Autodesk Inventor part; units mm, degrees
ref_plane "YZ Plane" through (0, 0, 0) normal (1, 0, 0) x (0, 1, 0)
ref_plane "XZ Plane" through (0, 0, 0) normal (0, 1, 0) x (-1, 0, 0)
ref_plane "XY Plane" through (0, 0, 0) normal (0, 0, 1) x (1, 0, 0)
sketch "Sketch1" plane through (0, 0, 0) normal (0, 0, 1) x (1, 0, 0)
  line L0 (-30, -85) -> (30, -85)
  line L1 (30, -85) -> (30, 85)
  line L2 (30, 85) -> (-30, 85)
  line L3 (-30, 85) -> (-30, -85)
  line L4 (-30, -85) -> (30, 85) construction
  line L5 (30, -85) -> (-30, 85) construction
  line L6 (-19, 19) -> (19, 19)
  line L7 (19, 19) -> (19, -19)
  line L8 (19, -19) -> (-19, -19)
  line L9 (-19, -19) -> (-19, 19)
  line L10 (-19, 19) -> (19, -19) construction
  line L11 (19, 19) -> (-19, -19) construction
  circle A0 centre (19, 19) radius 1.5875
  circle A1 centre (19, 19) radius 3
  circle A2 centre (-19, 19) radius 3
  circle A3 centre (-19, 19) radius 1.5875
  circle A4 centre (-19, -19) radius 3
  circle A5 centre (-19, -19) radius 1.5875
  circle A6 centre (19, -19) radius 3
  circle A7 centre (19, -19) radius 1.5875
  circle A8 centre (19, -35) radius 3
  circle A9 centre (19, -35) radius 1.5875
  circle A10 centre (-19, -35) radius 1.5875
  circle A11 centre (-19, -35) radius 3
  circle A12 centre (-19, -73) radius 3
  circle A13 centre (-19, -73) radius 1.5875
  circle A14 centre (19, -73) radius 3
  circle A15 centre (19, -73) radius 1.5875
  circle A16 centre (19, 73) radius 3
  circle A17 centre (19, 73) radius 1.5875
  circle A18 centre (-19, 73) radius 1.5875
  circle A19 centre (-19, 73) radius 3
  circle A20 centre (-19, 35) radius 3
  circle A21 centre (-19, 35) radius 1.5875
  circle A22 centre (19, 35) radius 3
  circle A23 centre (19, 35) radius 1.5875
  circle A24 centre (19, 19) radius 3
  circle A25 centre (19, 19) radius 1.5875
  circle A26 centre (-19, 19) radius 1.5875
  circle A27 centre (-19, 19) radius 3
  circle A28 centre (-19, -19) radius 3
  circle A29 centre (-19, -19) radius 1.5875
  circle A30 centre (19, -19) radius 3
  circle A31 centre (19, -19) radius 1.5875
  point P0 (0, 0)
  dimension "d0" = 170
  dimension "d1" = 60
  dimension "d2" = 38
  dimension "d3" = 38
  dimension "d6" = 6
  dimension "d7" = 3.175
  dimension "d10" = 360
  dimension "d14" = 54
  dimension "d17" = 54
extrude "Extrusion1" add sketch "Sketch1" along normal blind 3.2 contours L3 L2 L1 L0 | L6 A1 L7 A6 L8 A4 L9 A2
extrude "Extrusion2" add sketch "Sketch1" along normal blind 5 contours A3 L9 A2 L6 | L6 A2 L9 A3 | A1 L7 A0 L6 | L6 A0 L7 A1 | A4 L8 A5 L9 | L9 A5 L8 A4 | A6 L8 A7 L7 | L7 A7 L8 A6 | A8 | A11 | A12 | A14 | A16 | A19 | A20 | A22
sketch "Sketch2" plane through (0, 0, 3.2) normal (0, 0, 1) x (1, 0, 0)
  line L0 (-15.4, 31.4) -> (-0.6, 31.4)
  line L1 (-0.6, 31.4) -> (-0.6, 26.4)
  line L2 (-0.6, 26.4) -> (-15.4, 26.4)
  line L3 (-15.4, 26.4) -> (-15.4, 31.4)
  circle A0 centre (-19, 35) radius 1.5875
  line L4 (-19, 35) -> (-15.4, 31.4)
  line L5 (-19, 35) -> (-14, 35)
  line L6 (-30, 85) -> (-30, -85)
  line L7 (-30, 0) -> (-30, 23)
  line L8 (-15.4, -22.6) -> (-0.6, -22.6)
  line L9 (-0.6, -22.6) -> (-0.6, -27.6)
  line L10 (-0.6, -27.6) -> (-15.4, -27.6)
  line L11 (-15.4, -27.6) -> (-15.4, -22.6)
  line L12 (-15.4, -76.6) -> (-0.6, -76.6)
  line L13 (-0.6, -76.6) -> (-0.6, -81.6)
  line L14 (-0.6, -81.6) -> (-15.4, -81.6)
  line L15 (-15.4, -81.6) -> (-15.4, -76.6)
  line L16 (-14.2, 31.4) -> (-15.4, 30.2)
  line L17 (-8, 26.4) -> (-8, 31.4)
  line L18 (-0.6, 28.9) -> (-8, 28.9)
  line L19 (-1.8, 31.4) -> (-0.6, 30.2)
  line L20 (-14.2, 26.4) -> (-15.4, 27.6)
  line L21 (-1.8, 26.4) -> (-0.6, 27.6)
  line L22 (-14.2, -22.6) -> (-15.4, -23.8)
  line L23 (-1.8, -22.6) -> (-0.6, -23.8)
  line L24 (-1.8, -27.6) -> (-0.6, -26.4)
  line L25 (-14.2, -27.6) -> (-15.4, -26.4)
  line L26 (-14.2, -76.6) -> (-15.4, -77.8)
  line L27 (-1.8, -76.6) -> (-0.6, -77.8)
  line L28 (-1.8, -81.6) -> (-0.6, -80.4)
  line L29 (-14.2, -81.6) -> (-15.4, -80.4)
  point P0 (0, 0)
  point P1 (-15.4, -80.4)
  point P2 (-0.6, -80.4)
  point P3 (-0.6, -77.8)
  point P4 (-15.4, -77.8)
  point P5 (-15.4, -26.4)
  point P6 (-0.6, -26.4)
  point P7 (-0.6, -23.8)
  point P8 (-15.4, -23.8)
  point P9 (-15.4, 27.6)
  point P10 (-0.6, 27.6)
  point P11 (-0.6, 30.2)
  dimension "d24" = 5
  dimension "d25" = 45
  dimension "d26" = 14.8
  dimension "d27" = 5
  dimension "d31" = 54
  dimension "d38" = 3.6
  dimension "d39" = 135
  dimension "d40" = 1.2
  dimension "d43" = 54
extrude "Extrusion3" cut sketch "Sketch2" against normal blind 5 contours L0 L17 L2 L20 L3 L16 | L0 L19 L1 L18 L17 | L18 L1 L21 L2 L17 | L8 L23 L9 L24 L10 L25 L11 L22 | L12 L27 L13 L28 L14 L29 L15 L26
sketch "Sketch4" plane through (0, 0, 3.2) normal (0, 0, 1) x (1, 0, 0)
  line L0 (-30, 85) -> (-30, -85)
  line L1 (-30, -85) -> (30, -85)
  line L2 (30, -85) -> (30, -110)
  line L3 (30, -110) -> (-30, -110)
  line L4 (-30, -110) -> (-30, -85)
  point P0 (0, 0)
  dimension "d54" = 60
  dimension "d55" = 25
properties part number "BasePotencia" material "Gold"
Here's how the part is built. I have some questions about the finished solid (model axes, mm). A direction names the side the tool comes from. Coordinates: 2 decimals unless noted, no trailing zeros. Write each loop counter-clockwise with the first axis right and the second up, starting at its lowest first coordinate (ties: lowest second). Pieces come first, ordered by that corner, then holes.
1) If we section it at D-D (x = 3): List the corners of the cut face in (y, z) for me, plus the area to 3 significant figures.
Filled in:
outline: (-85, 0) - (85, 0) - (85, 3.2) - (-85, 3.2) - close
area: 544 mm2
2) Which directions (+Z, -Z, +X, -X, +Y, -Y) give clear straight access to the entire face, cutting with the end or side of a thin tool? Please do faces 4 (the face through (-18.27, -17.59, 2.46)), 5 (the face through (-21.21, 32.97, 4.09)).
Filled in:
face 4: +Z, -Z
face 5: +Z
3) If I drill on line 1 (Y direction, x = -10, z = 2.4); line 2 (X direction, y = 19, z = 3.3); line 3 (X direction, y = 73, z = 1.1), over which ranges is the centre line in solid material (lowest first)?
Filled in:
line 1: y = -85 to -81.6, -76.6 to -27.6, -22.6 to 26.4, 31.4 to 85
line 2: x = -22 to -20.59, -17.41 to -16, 16 to 17.41, 20.59 to 22
line 3: x = -30 to -20.59, -17.41 to 17.41, 20.59 to 30
4) If we section it at A-A (y = 19): List the corners of the cut face in (x, z) for me.
Filled in:
outline: (-30, 0) - (-20.59, 0) - (-20.59, 5) - (-22, 5) - (-22, 3.2) - (-30, 3.2) - close; (-17.41, 0) - (17.41, 0) - (17.41, 5) - (16, 5) - (16, 3.2) - (-16, 3.2) - (-16, 5) - (-17.41, 5) - close; (20.59, 0) - (30, 0) - (30, 3.2) - (22, 3.2) - (22, 5) - (20.59, 5) - close
5) Thinking about a two-plate mould opening in Y: for faces 1 (the face through (-18.15, -36.34, 2.46)), 2 (the face through (0, -85, 2)), 3 (the face through (30, -1, 2)), which applies, +Y half, -Y half, draft (parallel to the pull), parting line (faces both ways), or undercut?
Filled in:
face 1: undercut
face 2: -Y half
face 3: draft
6) If we section it at B-B (x = 19): Count the separate pieces of the cut face and the enclosed holes in it, plus the area to 3 significant figures.
Filled in:
separate pieces: 7
enclosed holes: 0
area: 514 mm2
